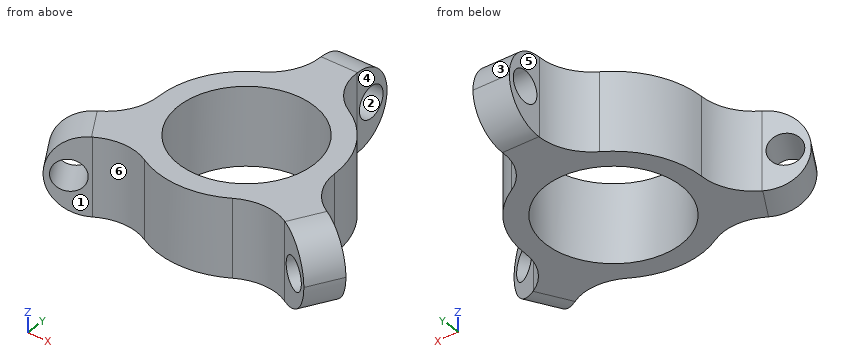
```python
from build123d import *

# Parameters (mm, degrees)
ESQUISSE1_R                  = 13
BOSS_EXTRU_1_DEPTH           = 15
CONG_1_R                     = 7.5
CONG_2_R                     = 7.5
CONG_3_R                     = 7.5
ENL_V_MAT_EXTRU_1_REACH      = 50.052
ESQUISSE2_R                  = 3
R_P_TITION_CIRCULAIRE1_COUNT = 3


with BuildPart() as part:
    # Esquisse1 → Boss.-Extru.1 (new body)
    with BuildSketch(Plane.XY):
        with BuildLine():
            Line((-3.5, 23.382685902), (-3.5, 31.041209697))
            Line((-3.5, 31.041209697), (3.5, 31.041209697))
            Line((3.5, 31.041209697), (3.5, 23.382685902))
            ThreePointArc((3.5, 23.382685902), (4.839745962, 18.382685902), (8.5, 14.722431864))
            ThreePointArc((8.5, 14.722431864), (14.722431864, 8.5), (17, 0))
            ThreePointArc((17, 0), (18.339745962, -5), (22, -8.660254038))
            Line((22, -8.660254038), (28.632476161, -12.489515935))
            Line((28.632476161, -12.489515935), (25.132476161, -18.551693762))
            Line((25.132476161, -18.551693762), (18.5, -14.722431864))
            ThreePointArc((18.5, -14.722431864), (13.5, -13.382685902), (8.5, -14.722431864))
            ThreePointArc((8.5, -14.722431864), (0, -17), (-8.5, -14.722431864))
            ThreePointArc((-8.5, -14.722431864), (-13.5, -13.382685902), (-18.5, -14.722431864))
            Line((-18.5, -14.722431864), (-25.132476161, -18.551693762))
            Line((-25.132476161, -18.551693762), (-28.632476161, -12.489515935))
            Line((-28.632476161, -12.489515935), (-22, -8.660254038))
            ThreePointArc((-22, -8.660254038), (-18.339745962, -5), (-17, 0))
            ThreePointArc((-17, 0), (-14.722431864, 8.5), (-8.5, 14.722431864))
            ThreePointArc((-8.5, 14.722431864), (-4.839745962, 18.382685902), (-3.5, 23.382685902))
        make_face()
        Circle(ESQUISSE1_R, mode=Mode.SUBTRACT)
    extrude(amount=BOSS_EXTRU_1_DEPTH)

    # Congé1
    cong_1_edges = [part.edges().sort_by_distance(p)[0] for p in [
        (0, 31.041209697, 0),
        (0, 31.041209697, 15),
    ]]
    fillet(cong_1_edges, radius=CONG_1_R - 0.0001)  # a hair under: the kernel refuses the full size

    # Congé2
    cong_2_edges = [part.edges().sort_by_distance(p)[0] for p in [
        (26.882476161, -15.520604848, 0),
        (26.882476161, -15.520604848, 15),
    ]]
    fillet(cong_2_edges, radius=CONG_2_R - 0.0001)  # a hair under: the kernel refuses the full size

    # Congé3
    cong_3_edges = [part.edges().sort_by_distance(p)[0] for p in [
        (-26.882476161, -15.520604848, 15),
        (-26.882476161, -15.520604848, 0),
    ]]
    fillet(cong_3_edges, radius=CONG_3_R - 0.0001)  # a hair under: the kernel refuses the full size

    # Esquisse2 → Enlèv. mat.-Extru.1 (cut, up to next)
    with BuildSketch(Plane(origin=(-1.75, -3.031088913, 0), x_dir=(0.8660254037844389, -0.4999999999999995, 0), z_dir=(-0.4999999999999995, -0.8660254037844389, 0)), mode=Mode.PRIVATE) as enl_v_mat_extru_1_sk1:
        with Locations((27.041209697, 7.5)):
            Circle(ESQUISSE2_R)
    enl_v_mat_extru_1_tool1 = extrude(enl_v_mat_extru_1_sk1.sketch, amount=-ENL_V_MAT_EXTRU_1_REACH, mode=Mode.PRIVATE) & part.part
    enl_v_mat_extru_1 = enl_v_mat_extru_1_tool1.solids().sort_by_distance((21.668375, -16.551694, 7.5))[0]
    add(enl_v_mat_extru_1, mode=Mode.SUBTRACT)

    # Répétition circulaire1: Enlèv. mat.-Extru.1 ×3 about axis
    r_p_tition_circulaire1_axis = Axis((0, 0, 15), (0, 0, -1))
    for i in range(1, R_P_TITION_CIRCULAIRE1_COUNT):
        add(enl_v_mat_extru_1.rotate(r_p_tition_circulaire1_axis, i * 360 / R_P_TITION_CIRCULAIRE1_COUNT), mode=Mode.SUBTRACT)


solid = part.part
```
Model file for the job. Use its own axes, mm. Face numbers are marked on the shaded views. A direction names the side the tool comes from. Coordinates: 2 decimals unless noted, no trailing zeros. Loops run counter-clockwise (first coordinate to the right, second up) from the corner with the lowest first, then second, coordinate; pieces in that order, holes last. Notation, with made-up numbers: (82, 18.5) - (104, 18.5) arc R21 ccw to (104, 55.5) - close; hole circle Ø7 at (81, 30.5). An arc over 180 degrees is marked (long way). Write item = value, one per line. Start each with the question number.
Item 1: Saw through at A-A, the plane x = 0. State how many separate pieces and enclosed holes the cut face has, then the cut area to 3 significant figures.
Item 2: 3-axis set-ups, long thin cutter, end or side, ignore diameter. For the marked faces 4, 5 and 6: which of +Z, -Z, +X, -X, +Y, -Y reach the whole face in a straight line?
Item 3: Saw through at D-D, the plane z = 1.5. List the corners of the cut face in (x, y), then the cut area to 3 significant figures.
Item 4: Saw through at C-C, the plane y = -6. List the corners of the cut face in (x, z).
Item 5: Wall check: probe 1 along Y at (x, z) = (0.5, 9); probe 2 along X at (y, z) = (23, 13.25); probe 3 along X at (y, z) = (-15.5, 5). Give the ranges that are in metal, low to high. Write a range as [from, to].
Item 6: Pull direction Z, two halves, no side cores. Call the marked faces 1, 2 and 3: +Z half, -Z half, draft (parallel to the pull), parting line (faces both ways), or undercut.
Item 7: Drop flat-ended pins along their axis: pin 1 Ø8.5 at (y, z) = (25.5, 5) entering from -X; pin 2 Ø2 at (y, z) = (5.5, 9.5) entering from -X; pin 3 Ø3 at (x, z) = (14, 6) entering from -Y. Give the stop position or say it passes through.
Answers:
q1.separate_pieces = 2
q1.enclosed_holes = 1
q1.area = 278 mm2
q2.face_4 = +Z, -Z, +X, +Y
q2.face_5 = +Z, -Z, -X, +Y
q2.face_6 = +Z, -Z, -Y
q3.outline = (-26.03, -10.99) - (-22.53, -17.05) - (-18.5, -14.72) arc R10 cw to (-8.5, -14.72) arc R17 ccw to (8.5, -14.72) arc R10 cw to (18.5, -14.72) - (22.53, -17.05) - (26.03, -10.99) - (22, -8.66) arc R10 cw to (17, 0) arc R17 ccw to (8.5, 14.72) arc R10 cw to (3.5, 23.38) - (3.5, 28.04) - (-3.5, 28.04) - (-3.5, 23.38) arc R10 cw to (-8.5, 14.72) arc R17 ccw to (-17, 0) arc R10 cw to (-22, -8.66) - close; hole circle Ø26 at (0, 0)
q3.area = 654 mm2
q4.outline = (-19, 0) - (-11.53, 0) - (-11.53, 15) - (-19, 15) - close; (11.53, 0) - (19, 0) - (19, 15) - (11.53, 15) - close
q5.probe_1 = [-16.99, -12.99], [12.99, 24.44], [29.64, 30.89]
q5.probe_2 = [-3.51, 3.51]
q5.probe_3 = [-26.4, -24.19], [-20.36, -19.85], [-6.98, 6.98], [19.85, 20.36], [24.19, 26.4]
q6.face_1 = draft
q6.face_2 = undercut
q6.face_3 = +Z half
q7.pin_1 = -3.73
q7.pin_2 = -16.39
q7.pin_3 = -13.58
